Could you check a few things on this drawing? It's one solid part, dimensions in mm from its lowest x, y, z. Coordinates: 2 decimals unless noted, no trailing zeros. Write each loop counter-clockwise with the first axis right and the second up, starting at its lowest first coordinate (ties: lowest second). Pieces come first, ordered by that corner, then holes. Notation, with made-up numbers: (77.5, 0) - (104.5, 0) arc R25 cw to (104.5, 32) - close; hole circle Ø8 at (43.5, 67.5). An arc over 180 degrees is marked (long way). Use one line per item in the form item = value. Start each with the question number.
(1) If we section it at B-B on y = 12: Please give me the cut outline in (x, z) (1 decimal).
(2) If we section it at C-C on z = 1.1: Please give me the cut outline in (x, y).
(3) If we section it at D-D on y = 4.5: Please give me the cut outline in (x, z).
(4) If I drill on probe 1 along X at (y, z) = (1.9, 2.5); probe 2 along Z at (x, y) = (26, 1.15); probe 3 along X at (y, z) = (13.25, 3.8), over which ranges is the centre line in solid material (lowest first)? Write a range as from..to.
(5) If we section it at A-A on x = 15: Please give me the cut outline in (y, z).
(6) Thinking about a two-plate mould opening in Y: for the marked faces 1, 2, 3 and 4, which applies, pulls with the +Y half, pulls with the -Y half, needs draft (parallel to the pull), parting line crosses it, or undercut?
(7) For pin 1 Ø2 at (x, z) = (4, 2.5) entering from +Y, with a flat end and sliding along its axis, tell me the tip position at first contact or that it passes through.
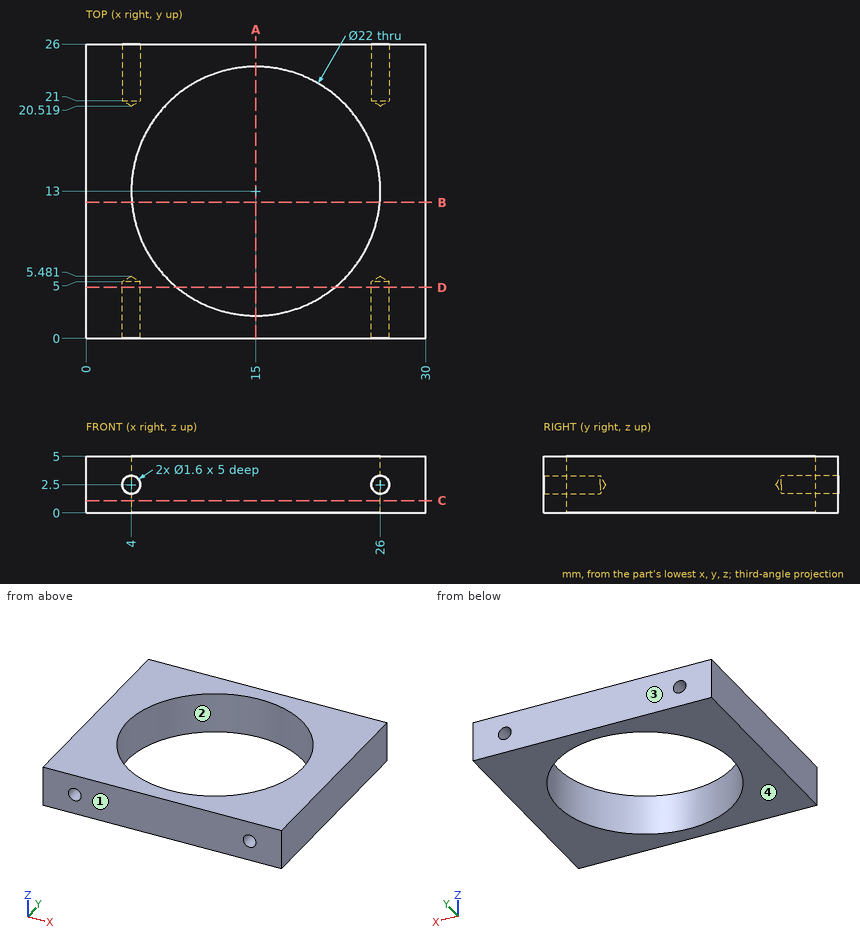
Reported:
q1.outline = (0, 0) - (4, 0) - (4, 5) - (0, 5) - close; (26, 0) - (30, 0) - (30, 5) - (26, 5) - close
q2.outline = (0, 0) - (30, 0) - (30, 26) - (0, 26) - close; hole circle Ø22 at (15, 13)
q3.outline = (0, 0) - (8.02, 0) - (8.02, 5) - (0, 5) - close; (21.98, 0) - (30, 0) - (30, 5) - (21.98, 5) - close; hole circle Ø1.6 at (4, 2.5); hole circle Ø1.6 at (26, 2.5)
q4.probe_1 = 0..3.2, 4.8..25.2, 26.8..30
q4.probe_2 = 0..1.7, 3.3..5
q4.probe_3 = 0..4, 26..30
q5.outline = (0, 0) - (2, 0) - (2, 5) - (0, 5) - close; (24, 0) - (26, 0) - (26, 5) - (24, 5) - close
q6.face_1 = pulls with the -Y half
q6.face_2 = undercut
q6.face_3 = pulls with the +Y half
q6.face_4 = needs draft
q7.pin_1 = 26
